```python
from build123d import *

# Parameters (mm, degrees)
SKETCH1_W                   = 150
SKETCH1_H                   = 150
BOSS_EXTRUDE1_DEPTH         = 15
SKETCH2_R                   = 12.5
CUT_EXTRUDE1_DEPTH          = 11
SKETCH3_R                   = 4
CUT_EXTRUDE2_DEPTH          = 107.6348911
SKETCH4_R                   = 50
CUT_EXTRUDE3_DEPTH          = 2
M3_TAPPED_HOLE1_D           = 2.5
M3_TAPPED_HOLE1_DEPTH       = 7.5
M3_TAPPED_HOLE1_CSINK_D     = 3.05
M3_TAPPED_HOLE1_CSINK_ANGLE = 90
M3_TAPPED_HOLE1_TIP         = 0.751075774
CHAMFER2_SIZE               = 5
CHAMFER1_SIZE               = 1


with BuildPart() as part:
    # Sketch1 → Boss-Extrude1 (new body)
    with BuildSketch(Plane(origin=(0, 0, 0), x_dir=(1, 0, 0), z_dir=(0, 1, 0))):
        Rectangle(SKETCH1_W, SKETCH1_H)
    extrude(amount=BOSS_EXTRUDE1_DEPTH)

    # Sketch2 → Cut-Extrude1 (cut)
    with BuildSketch(Plane(origin=(0, 0, 0), x_dir=(-1, 0, 0), z_dir=(0, -1, 0))):
        with Locations(Location((0, 0, 0), (0, 0, 90))):
            Circle(SKETCH2_R)
    extrude(amount=-CUT_EXTRUDE1_DEPTH, mode=Mode.SUBTRACT)

    # Sketch3 → Cut-Extrude2 (cut, through all)
    with BuildSketch(Plane(origin=(0, 11, 0), x_dir=(-1, 0, 0), z_dir=(0, -1, 0))):
        with Locations(Location((0, 0, 0), (0, 0, 90))):
            Circle(SKETCH3_R)
    extrude(amount=-CUT_EXTRUDE2_DEPTH, mode=Mode.SUBTRACT)

    # Sketch4 → Cut-Extrude3 (cut)
    with BuildSketch(Plane(origin=(0, 15, 0), x_dir=(1, 0, 0), z_dir=(0, 1, 0))):
        with Locations(Location((0, 0, 0), (0, 0, 270))):
            Circle(SKETCH4_R)
    extrude(amount=-CUT_EXTRUDE3_DEPTH, mode=Mode.SUBTRACT)

    # M3 Tapped Hole1
    with Locations(Plane(origin=(8.25, 11, 0), x_dir=(0, 0, -1), z_dir=(0, -1, 0))):
        with Locations((0, 0), (0, -16.5)):
            CounterSinkHole(M3_TAPPED_HOLE1_D / 2, M3_TAPPED_HOLE1_CSINK_D / 2, depth=M3_TAPPED_HOLE1_DEPTH, counter_sink_angle=M3_TAPPED_HOLE1_CSINK_ANGLE)
            with Locations((0, 0, -(M3_TAPPED_HOLE1_DEPTH + M3_TAPPED_HOLE1_TIP / 2))):  # 118° drill point
                Cone(0, M3_TAPPED_HOLE1_D / 2, M3_TAPPED_HOLE1_TIP, mode=Mode.SUBTRACT)

    # Chamfer2
    chamfer2_edges = [part.edges().sort_by_distance(p)[0] for p in [
        (75, 7.5, 75),
        (-75, 7.5, 75),
        (-75, 7.5, -75),
        (75, 7.5, -75),
    ]]
    chamfer(chamfer2_edges, length=CHAMFER2_SIZE)

    # Chamfer1
    chamfer1_edges = [part.edges().sort_by_distance(p)[0] for p in [
        (0, 15, -50),
        (0, 15, -75),
        (75, 15, 0),
        (-75, 15, 0),
        (0, 15, 75),
        (-72.5, 15, -72.5),
        (-72.5, 15, 72.5),
        (72.5, 15, 72.5),
        (72.5, 15, -72.5),
    ]]
    chamfer(chamfer1_edges, length=CHAMFER1_SIZE)


solid = part.part
```
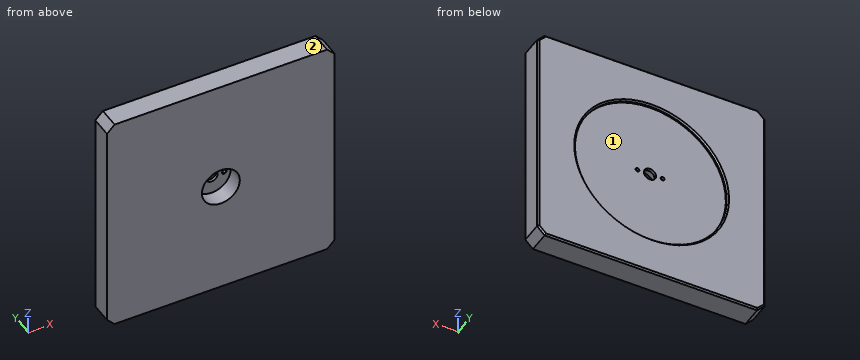
Verification items for the finished model (mm, model axes). Face numbers are marked on the shaded views. Coordinates: 2 decimals unless noted, no trailing zeros. Write each loop counter-clockwise with the first axis right and the second up, starting at its lowest first coordinate (ties: lowest second). Pieces come first, ordered by that corner, then holes. Notation, with made-up numbers: (29, 81) - (39, 81) arc R26 cw to (39, 113) - close; hole circle Ø7 at (-23.75, -1). An arc over 180 degrees is marked (long way). Write item = value, one per line.
Q1. Material ranges on L1, parallel to X at y = 12.15, z = 0; L2, parallel to X at y = 13.5, z = 0; L3, parallel to Z at x = -8.25, y = 12.55, recorded low to high. Write a range as from..to.
Answer:
L1 = -75..-9.5, -7..-4, 4..7, 9.5..75
L2 = -75..-50, 50..75
L3 = -75..-1.25, 1.25..75
Q2. Cross-section at B-B (y = 8). Enter the section's corners in (x, z), plus the area to 3 significant figures.
Answer:
outline = (-75, -70) - (-70, -75) - (70, -75) - (75, -70) - (75, 70) - (70, 75) - (-70, 75) - (-75, 70) - close; hole circle Ø25 at (0, 0)
area = 22,000 mm²
Q3. Cross-section at A-A (x = 0). Enter the section's corners in (y, z).
Answer:
outline = (0, -75) - (14, -75) - (15, -74) - (15, -51) - (14, -50) - (13, -50) - (13, -4) - (11, -4) - (11, -12.5) - (0, -12.5) - close; (0, 12.5) - (11, 12.5) - (11, 4) - (13, 4) - (13, 50) - (14, 50) - (15, 51) - (15, 74) - (14, 75) - (0, 75) - close
Q4. Mould release check, pull along X, two halves, no side actions. Record for the marked faces 1 and 2: released by +X, released by -X, zero draft, split by the parting line, or undercut.
Answer:
face_1 = undercut
face_2 = zero draft
Q5. Go/stop test with flat-tipped pins: pin 1 Ø3 at (x, z) = (-8.25, 0) entering from -Y (3 decimals); pin 2 Ø20 at (x, z) = (0, 0) entering from +Y; pin 3 Ø2 at (x, z) = (8.25, 0) entering from -Y. Record where each tip stops, or that it passes through.
Answer:
pin_1 = 11.025
pin_2 = 13
pin_3 = through
